from build123d import *

# Parameters (mm, degrees)
BOSS_EXTRUDE1_DEPTH = 10
FILLET1_R           = 10
FILLET2_R           = 10
FILLET3_R           = 3


with BuildPart() as part:
    # Sketch1 → Boss-Extrude1 (new body)
    with BuildSketch(Plane.XY):
        with BuildLine():
            Line((-94.626197475, -89.797589363), (-83.792, -85.26796022))
            ThreePointArc((-83.792, -85.26796022), (-95.098975753, -72.442453815), (-104.460674711, -58.135116263))
            Line((-104.460674711, -58.135116263), (-18.296393823, -17.036489459))
            ThreePointArc((-18.296393823, -17.036489459), (0, -25), (18.296393823, -17.036489459))
            Line((18.296393823, -17.036489459), (104.460674711, -58.135116263))
            ThreePointArc((104.460674711, -58.135116263), (95.098975753, -72.442453815), (83.792, -85.26796022))
            Line((83.792, -85.26796022), (88.131779474, -96.179591135))
            ThreePointArc((88.131779474, -96.179591135), (107.052618298, -74.548381737), (120.777959535, -49.299176408))
            Line((120.777959535, -49.299176408), (24.754108024, -3.497732969))
            ThreePointArc((24.754108024, -3.497732969), (0, 25), (-24.754108024, -3.497732969))
            Line((-24.754108024, -3.497732969), (-120.777959535, -49.299176408))
            ThreePointArc((-120.777959535, -49.299176408), (-109.589087401, -70.766914774), (-94.626197475, -89.797589363))
        make_face()
        with BuildLine():
            ThreePointArc((4.275251792, 11.74615776), (0, -12.5), (-4.275251792, 11.74615776))
            Line((-4.275251792, 11.74615776), (0, 0))
            Line((0, 0), (4.275251792, 11.74615776))
        make_face(mode=Mode.SUBTRACT)
    extrude(amount=BOSS_EXTRUDE1_DEPTH)

    # Fillet1
    fillet1_edges = [part.edges().sort_by_distance(p)[0] for p in [
        (-24.754108024, -3.497732969, 5),
        (24.754108024, -3.497732969, 5),
        (18.296393823, -17.036489459, 5),
        (-18.296393823, -17.036489459, 5),
    ]]
    fillet(fillet1_edges, radius=FILLET1_R)

    # Fillet2
    fillet2_edges = [part.edges().sort_by_distance(p)[0] for p in [
        (-104.460674711, -58.135116263, 5),
        (-120.777959535, -49.299176408, 5),
        (120.777959535, -49.299176408, 5),
        (104.460674711, -58.135116263, 5),
    ]]
    fillet(fillet2_edges, radius=FILLET2_R)

    # Fillet3
    fillet3_edges = [part.edges().sort_by_distance(p)[0] for p in [
        (4.275251792, 11.74615776, 5),
        (-4.275251792, 11.74615776, 5),
    ]]
    fillet(fillet3_edges, radius=FILLET3_R)


solid = part.part
The model under review builds one solid part; all positions refer to its coordinate system, in mm. A direction names the side the tool comes from. Give positions to 0.01 mm unless a question says otherwise; leave off trailing zeros. Loops run counter-clockwise (first coordinate to the right, second up) from the corner with the lowest first, then second, coordinate; pieces in that order, holes last. Notation, with made-up numbers: (-19, -31) -> (-9, -31) arc R30 cw to (-9, 2) -> close; hole circle Ø9 at (59.5, 45.5). An arc over 180 degrees is marked (long way). Answer as a JSON object with one key per item and string values. Group by question number.
Q1. Draft analysis for pull direction X (two halves, no side actions). For faces 4 (the cylindrical face through (-106.89, -74.78, 4.93)), 5 (the cylindrical face through (-19.11, -18.87, 5.07)), 6 (the cylindrical face through (117.042, -50.756, 5.07)), state which applies: pulls with the +X half, pulls with the -X half, needs draft (parallel to the pull), parting line crosses it, or undercut.
Q2. Tool access review of faces 1 (the cylindrical face through (-117.042, -50.756, 5.07)), 2 (the cylindrical face through (99.767, -59.897, 5.07)), 3 (the flat face through (-89.285, -87.564, 4.93)): name each direction out of +Z, -Z, +X, -X, +Y, -Y from which nothing blocks a thin tool from reaching the whole face with its end or side.
Q3. Take a section at B-B (y = -48.5). Write out the cut boundary in (x, z).
Q4. Take a section at D-D (x = 52). Write out the cut boundary in (y, z).
Q5. Take a section at C-C (y = -78). Write out the cut boundary in (x, z).
Q6. Insertion check: pin 1 (6 mm diameter, centred on x = 64, z = 3.5, fed in from -Y); pin 2 (3 mm diameter, centred on x = 69.5, z = 8, fed in from +Y); pin 3 (1 mm diameter, centred on y = -30, z = 6.5, fed in from -X) (3 decimals). Each pin has a flat end and moves straight along its axis. Give the tip position at first contact, or say it passes through.
Q7. Take a section at A-A (z = 2). Write out the cut boundary in (x, y), plus the area to 3 significant figures.
Q8. Wall thickness on line 1 along X through (y, z) = (0.5, 4.75); line 2 along Y through (x, z) = (92, 7.25); line 3 along X through (y, z) = (2.5, 5.5): over which ranges is each line inside the solid? List them lowest first.
Answer below:
{
 "1": {"face 4": "pulls with the -X half", "face 5": "undercut", "face 6": "pulls with the +X half"},
 "2": {"face 1": "+Z, -Z, -X", "face 2": "+Z, -Z", "face 3": "+Z, -Z, -Y"},
 "3": {"outline": "(-115.9, 0) -> (-84.26, 0) -> (-84.26, 10) -> (-115.9, 10) -> close; (84.26, 0) -> (115.9, 0) -> (115.9, 10) -> (84.26, 10) -> close"},
 "4": {"outline": "(-33.11, 0) -> (-16.49, 0) -> (-16.49, 10) -> (-33.11, 10) -> close"},
 "5": {"outline": "(-104.56, 0) -> (-90.6, 0) -> (-90.6, 10) -> (-104.56, 10) -> close; (90.6, 0) -> (104.56, 0) -> (104.56, 10) -> (90.6, 10) -> close"},
 "6": {"pin 1": "stops at y = -40.27", "pin 2": "stops at y = -24.13", "pin 3": "stops at x = -81.365"},
 "7": {"outline": "(-116.55, -58.59) arc R130.45 ccw to (-94.63, -89.8) -> (-83.79, -85.27) arc R119.55 cw to (-98.29, -68.04) arc R10 cw to (-94.38, -53.33) -> (-24.13, -19.82) arc R10 cw to (-14.16, -20.6) arc R25 ccw to (14.16, -20.6) arc R10 cw to (24.13, -19.82) -> (94.38, -53.33) arc R10 cw to (98.29, -68.04) arc R119.55 cw to (83.79, -85.27) -> (88.13, -96.18) arc R130.45 ccw to (116.55, -58.59) arc R10 ccw to (111.92, -45.08) -> (30.59, -6.28) arc R10 cw to (24.92, 1.96) arc R25 ccw to (-24.92, 1.96) arc R10 cw to (-30.59, -6.28) -> (-111.92, -45.08) arc R10 ccw to start; hole (-7.77, 9.8) arc R12.5 ccw (long way) to (7.77, 9.8) arc R3 ccw to (3.08, 8.47) -> (0, 0) -> (-3.08, 8.47) arc R3 ccw to start", "area": "5,540 mm2"},
 "8": {"line 1": "x = -25.15 to -12.49, -0.18 to 0.18, 12.49 to 25.15", "line 2": "y = -92.49 to -76.34, -52.19 to -35.57", "line 3": "x = -24.87 to -12.25, -0.91 to 0.91, 12.25 to 24.87"}
}
